```python
from build123d import *

# Parameters (mm, degrees)
F0_W      = 114.3
F0_H      = 5.08
F1_DEPTH  = 158.75
F2_W      = 12.7
F2_H      = 317.5
F3_DEPTH  = 127
F4_R      = 6.35
F5_DEPTH  = 5.08
F6_R      = 6.35
F7_DEPTH  = 5.08
F9_R      = 25.4
F10_DEPTH = 281.94
F11_R     = 6.35
F12_DEPTH = 327.66
F13_R     = 6.35
F14_DEPTH = 322.581


with BuildPart() as f1:
    # F0 (on Right) → F1 (new body, symmetric)
    with BuildSketch(Plane.YZ):
        Rectangle(F0_W, F0_H)
    extrude(amount=F1_DEPTH, both=True)

    # F2 (on face) → F3 (join)
    with BuildSketch(Plane.XY.offset(2.54)):
        with Locations((152.4, 101.6)):
            Rectangle(F2_W, F2_H)
        with Locations((-152.4, 101.6)):
            Rectangle(F2_W, F2_H)
    extrude(amount=F3_DEPTH)

    # F4 (on face) → F5 (join)
    with BuildSketch(Plane.YZ.offset(-146.05)):
        with BuildLine():
            Line((-38.1, 91.44), (-63.5, 91.44))
            ThreePointArc((-63.5, 91.44), (-82.55, 72.39), (-63.5, 53.34))
            Line((-63.5, 53.34), (-38.1, 53.34))
            Line((-38.1, 53.34), (-38.1, 91.44))
        make_face()
        with Locations((-71.12, 72.39)):
            Circle(F4_R, mode=Mode.SUBTRACT)
    extrude(amount=F5_DEPTH)

    # F6 (on face) → F7 (join)
    with BuildSketch(Plane(origin=(-158.75, 0, 0), x_dir=(0, -1, 0), z_dir=(-1, 0, 0))):
        with BuildLine():
            Line((63.5, 91.44), (38.1, 91.44))
            Line((38.1, 91.44), (38.1, 53.34))
            Line((38.1, 53.34), (63.5, 53.34))
            ThreePointArc((63.5, 53.34), (82.55, 72.39), (63.5, 91.44))
        make_face()
        with Locations((71.12, 72.39)):
            Circle(F6_R, mode=Mode.SUBTRACT)
    extrude(amount=F7_DEPTH)

    # F8: F1 across plane


with BuildPart() as f1_1:
    add(f1.part)
    add(f1.part.mirror(Plane.YZ))

    # F9 (on face) → F10 (join)
    with BuildSketch(Plane.YZ.offset(-140.97)):
        with Locations((-71.12, 72.39)):
            Circle(F9_R)
    extrude(amount=F10_DEPTH)

    # F11 (on face) → F12 (cut)
    with BuildSketch(Plane.YZ.offset(163.83)):
        with Locations((-71.12, 72.39)):
            Circle(F11_R)
    extrude(amount=-F12_DEPTH, mode=Mode.SUBTRACT)

    # F13 (on face) → F14 (cut, through all)
    with BuildSketch(Plane.YZ.offset(158.75)):
        with Locations((222.25, 97.79)):
            Circle(F13_R)
    extrude(amount=-F14_DEPTH, mode=Mode.SUBTRACT)


solid = f1_1.part
```
Can you work these out from the model? Positions are in its coordinate system, mm. A direction names the side the tool comes from. Give positions to 0.01 mm unless a question says otherwise; leave off trailing zeros. Order: outer loops, then holes, each group sorted by start corner. A loop starts at its lowest first (then second) coordinate and runs counter-clockwise, first axis right, second up. Notation, with made-up numbers: M 44,84 L 57,84 A19 cw 57,114 Z; hole C 50.5,40.25 d1. An arc over 180 degrees is marked long. Write item = value, one per line. Start each with the question number.
Q1. For faces 4 (the flat face through (-152, 160, 2.54)), 5 (the flat face through (-158.75, -64, 73)), 6 (the cylindrical face through (161.254, -82.545, 71.971)), which set-ups out of +Z, -Z, +X, -X, +Y, -Y let a thin tool reach every point of the face, with its end or its side?
Q2. Suppose I cut it at C-C (x = 75.5). Write out the boundary of the cut face in (y, z), plus the area to 3 significant figures.
Q3. Will these pins go through, and if not, where does the flat tip stop? pin 1 Ø12 at (x, z) = (-105.5, 94) entering from -Y; pin 2 Ø10 at (y, z) = (224.5, 25.5) entering from +X; pin 3 Ø4 at (x, y) = (155, 156.5) entering from -Z.
Q4. We'd pull the mould along Y, two halves only. Please class faces 1 (the cylindrical face through (152.489, 225.18, 92.156)), 2 (the flat face through (2, -1, 2.54)), 3 (the flat face through (-1, -57.15, 0)): pulls with the +Y half, pulls with the -Y half, needs draft (parallel to the pull), parting line crosses it, or undercut.
Q5. I need wall thicknesses on probe 1 along X at (y, z) = (-74, 79); probe 2 along X at (y, z) = (231.5, 121); probe 3 along Z at (x, y) = (27, -71.12). Which ranges of each line are inside material? Lowest first, please. Write a range as [from, to].
Q6. Suppose I cut it at D-D (y = -34). Write out the boundary of the cut face in (x, z).
Q7. Suppose I cut it at A-A (y = 222.25). Write out the boundary of the cut face in (x, z), plus the area to 3 significant figures.
Q8. Suppose I cut it at B-B (y = 71). Write out the boundary of the cut face in (x, z).
Check result:
q1.face_4 = -Z, +X, -X, +Y
q1.face_5 = +Z, -Z, -Y
q1.face_6 = +X, -Y
q2.outline = C -71.12,72.39 d50.8; M -57.15,-2.54 L 57.15,-2.54 L 57.15,2.54 L -57.15,2.54 Z; hole C -71.12,72.39 d12.7
q2.area = 2,480 mm2
q3.pin_1 = -91.16
q3.pin_2 = 158.75
q3.pin_3 = 2.54
q4.face_1 = undercut
q4.face_2 = needs draft
q4.face_3 = pulls with the -Y half
q5.probe_1 = [-163.83, -158.75], [-146.05, 146.05], [158.75, 163.83]
q5.probe_2 = [-158.75, -146.05], [146.05, 158.75]
q5.probe_3 = [46.99, 66.04], [78.74, 97.79]
q6.outline = M -158.75,-2.54 L 158.75,-2.54 L 158.75,129.54 L 146.05,129.54 L 146.05,2.54 L -146.05,2.54 L -146.05,129.54 L -158.75,129.54 Z
q7.outline = M -158.75,2.54 L -146.05,2.54 L -146.05,91.44 L -158.75,91.44 Z; M -158.75,104.14 L -146.05,104.14 L -146.05,129.54 L -158.75,129.54 Z; M 146.05,2.54 L 158.75,2.54 L 158.75,91.44 L 146.05,91.44 Z; M 146.05,104.14 L 158.75,104.14 L 158.75,129.54 L 146.05,129.54 Z
q7.area = 2,900 mm2
q8.outline = M -158.75,2.54 L -146.05,2.54 L -146.05,129.54 L -158.75,129.54 Z; M 146.05,2.54 L 158.75,2.54 L 158.75,129.54 L 146.05,129.54 Z
